Input: part model. Units: mm. Frame: model coordinates. A direction names the side the tool comes from. Round coordinates to 2 decimals unless told otherwise and drop trailing zeros. Loops run counter-clockwise (first coordinate to the right, second up) from the corner with the lowest first, then second, coordinate; pieces in that order, holes last. Notation, with made-up numbers: (0, -16.75) - (55, -16.75) arc R30 cw to (55, 19.25) - close; hole circle Ø11 at (76, -12.75). An arc over 180 degrees is marked (long way). Write each question's results on one line, items separated by ' | '.
from build123d import *

# Parameters (mm, degrees)
F0_W      = 121.2779134512
F0_H      = 37.155687809
F1_DEPTH  = 100
F2_DEPTH  = 25
F3_DEPTH  = 15
F4_W      = 65.5741617084
F4_H      = 89.4537195563
F5_DEPTH  = 1200
F7_W      = 45.3369794413
F7_H      = 69.372177124
F8_DEPTH  = 40
F9_W      = 45.3369794413
F9_H      = 34.686088562
F10_DEPTH = 25


with BuildPart() as f1:
    # F0 (on Top) → F1 (new body)
    with BuildSketch(Plane.XY):
        with Locations((-60.6389567256, -18.5778439045)):
            Rectangle(F0_W, F0_H)
    extrude(amount=F1_DEPTH)

    # F2 (add): a face of the model
    f2_faces = [f1.faces().sort_by_distance(p)[0] for p in [
        (-60.6389567256, -37.155687809, 50),
    ]]
    extrude(f2_faces, amount=F2_DEPTH)

    # F3 (add): a face of the model
    f3_faces = [f1.faces().sort_by_distance(p)[0] for p in [
        (-60.6389567256, -62.155687809, 50),
    ]]
    extrude(f3_faces, amount=F3_DEPTH)

    # F4 (on face) → F5 (cut)
    with BuildSketch(Plane.XZ.offset(77.155687809)):
        with Locations((-60.1045750082, 44.7268597782)):
            Rectangle(F4_W, F4_H)
    extrude(amount=-F5_DEPTH, mode=Mode.SUBTRACT)

    # F7 (on face) → F8 (join)
    with BuildSketch(Plane.YZ):
        with Locations((-37.7225787379, 34.686088562)):
            Rectangle(F7_W, F7_H)
    extrude(amount=F8_DEPTH)

    # F9 (on face) → F10 (join)
    with BuildSketch(Plane.YZ.offset(40)):
        with Locations((-37.7225787379, 17.343044281)):
            Rectangle(F9_W, F9_H)
    extrude(amount=F10_DEPTH)


solid = f1.part
1. Section query D-D, the plane x = 20.5. Output: boundary loops of the cut face in (y, z), plus the area to 3 significant figures.
Answer:
outline: (-60.39, 0) - (-15.05, 0) - (-15.05, 69.37) - (-60.39, 69.37) - close | area: 3,150 mm^2
2. Mould query, pull axis X, two halves, no side actions, for faces 1 (the flat face through (40, -38, 52)), 2 (the flat face through (20, -38, 69.372)), 3 (the flat face through (-27.317, -39, 44)). Classes: pulls with the +X half, pulls with the -X half, needs draft (parallel to the pull), parting line crosses it, or undercut.
Answer:
face 1: pulls with the +X half | face 2: needs draft | face 3: undercut
3. Section query C-C, the plane z = 38.5. Output: boundary loops of the cut face in (x, y), plus the area to 3 significant figures.
Answer:
outline: (-121.28, -77.16) - (-92.89, -77.16) - (-92.89, 0) - (-121.28, 0) - close; (-27.32, -77.16) - (0, -77.16) - (0, -60.39) - (40, -60.39) - (40, -15.05) - (0, -15.05) - (0, 0) - (-27.32, 0) - close | area: 6,110 mm^2
4. Line query: line 1 (X direction, y = -55, z = 29); line 2 (X direction, y = -70, z = 27.5); line 3 (Z direction, x = -90, y = -61). Output: solid intervals per line, ascending. Write a range as [from, to].
Answer:
line 1: [-121.28, -92.89], [-27.32, 65] | line 2: [-121.28, -92.89], [-27.32, 0] | line 3: [89.45, 100]
5. Section query A-A, the plane z = 28.5. Output: boundary loops of the cut face in (x, y), plus the area to 3 significant figures.
Answer:
outline: (-121.28, -77.16) - (-92.89, -77.16) - (-92.89, 0) - (-121.28, 0) - close; (-27.32, -77.16) - (0, -77.16) - (0, -60.39) - (65, -60.39) - (65, -15.05) - (0, -15.05) - (0, 0) - (-27.32, 0) - close | area: 7,240 mm^2
6. Section query B-B, the plane y = -31.5. Output: boundary loops of the cut face in (x, z), plus the area to 3 significant figures.
Answer:
outline: (-121.28, 0) - (-92.89, 0) - (-92.89, 89.45) - (-27.32, 89.45) - (-27.32, 0) - (65, 0) - (65, 34.69) - (40, 34.69) - (40, 69.37) - (0, 69.37) - (0, 100) - (-121.28, 100) - close | area: 9,900 mm^2
7. Set-up query: faces 4 (the flat face through (-61, -39, 89.454)), 5 (the flat face through (25, -60.391, 34)), 6 (the flat face through (52, -38, 34.686)). Return all of +Z, -Z, +X, -X, +Y, -Y with unobstructed straight access to the full face (end or side cutting, diameter ignored); none if empty.
Answer:
face 4: -Z, +Y, -Y | face 5: +Z, -Z, +X, -Y | face 6: +Z, +X, +Y, -Y
8. Contact query for flat-ended pins moving along their axis: pin 1 (10 mm diameter, centred on y = -62.5, z = 33.5, fed in from +X); pin 2 (5 mm diameter, centred on x = 5, y = -58, fed in from +Z); pin 3 (1 mm diameter, centred on y = -15.5, z = 58.5, fed in from +X); pin 4 (7.5 mm diameter, centred on x = 52.5, y = -49, fed in from +Z). Output: stop coordinate, or through.
Answer:
pin 1: x = 65 | pin 2: z = 69.37 | pin 3: x = 40 | pin 4: z = 34.69
